The listing builds one solid part. Answer for the finished solid, in the listing's coordinates (mm). Face numbers are marked on the shaded views. A direction names the side the tool comes from. Round coordinates to 2 decimals unless told otherwise and drop trailing zeros. Loops run counter-clockwise (first coordinate to the right, second up) from the corner with the lowest first, then second, coordinate; pieces in that order, holes last. Notation, with made-up numbers: (65, -37) -> (105, -37) arc R6 cw to (105, -27) -> close; hole circle Ø5 at (59.25, 89.5). An arc over 180 degrees is marked (long way). Write each question's results on one line, items separated by ' | '. Start each with the question number.
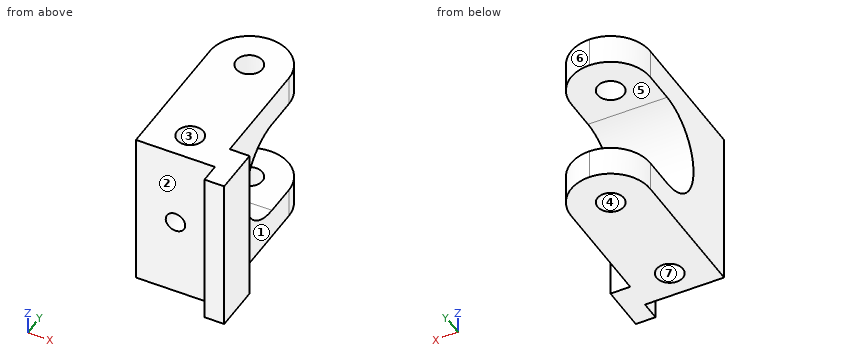
Autodesk Inventor part; units mm, degrees
ref_plane "YZ Plane" through (0, 0, 0) normal (1, 0, 0) x (0, 1, 0)
ref_plane "XZ Plane" through (0, 0, 0) normal (0, 1, 0) x (-1, 0, 0)
ref_plane "XY Plane" through (0, 0, 0) normal (0, 0, 1) x (1, 0, 0)
sketch "草圖1" plane through (0, 0, 0) normal (1, 0, 0) x (0, 1, 0)
  arc A0 (0, 12.5) -> (0, -12.5) centre (0, 0) ccw
  line L0 (-27, 0) -> (-27, -20)
  line L1 (-27, -20) -> (18, -20)
  line L2 (18, 20) -> (-27, 20)
  line L3 (-27, 20) -> (-27, 0)
  line L4 (0, 12.5) -> (18, 12.5)
  line L5 (18, -12.5) -> (0, -12.5)
  line L6 (18, -12.5) -> (18, -20)
  line L7 (18, 12.5) -> (18, 20)
  dimension "d5" = 25
  dimension "d12" = 18
  dimension "d13" = 45
  dimension "d15" = 40
  dimension "d16" = 45
  dimension "d17" = 7.5
  dimension "d18" = 7.5
  dimension "d19" = 18
extrude "擠出1" add sketch "草圖1" along normal mid plane 20
sketch "草圖2" plane through (-10, -27, 20) normal (0, 0, 1) x (1, 0, 0)
  line L0 (20, 0) -> (20, 45)
  line L1 (20, 0) -> (20, 7)
  line L2 (20, 7) -> (25, 7)
  line L3 (25, 7) -> (25, 0)
  line L4 (25, 0) -> (25, -5)
  line L5 (25, -5) -> (20, -5)
  line L6 (0, 0) -> (20, 0)
  line L7 (20, -5) -> (20, 0)
  point P0 (10, 27)
  dimension "d22" = 7
  dimension "d23" = 5
  dimension "d24" = 5
extrude "擠出2" add sketch "草圖2" against normal up to surface (40 mm away)
fillet "圓角1" radius 10 4 edges at (10, 18, 16.25) (-10, 18, 16.25) (10, 18, -16.25) (-10, 18, -16.25)
sketch "草圖3" plane through (10, -32, 20) normal (0, 0, 1) x (1, 0, 0)
  line L0 (-20, 5) -> (0, 5)
  point P0 (-10, 32)
  point P1 (-10, 40)
  dimension "d30" = 35
hole "孔1" at (0, 8, 20) direction (0, 0, -1) diameter 6.647 end through all
sketch "草圖4" plane through (10, -32, 20) normal (0, 0, 1) x (1, 0, 0)
  line L0 (-20, 5) -> (0, 5)
  point P0 (-10, 32)
  point P1 (-10, 12)
  dimension "d38" = 7
hole "孔2" at (0, -20, 20) direction (0, 0, -1) diameter 6.647 depth 12 tip angle 118
mirror "鏡射1" about plane through (0, 0, 0) normal (0, 0, 1) of "孔2"
sketch "草圖5" plane through (-10, -27, -20) normal (0, -1, 0) x (1, 0, 0)
  point P0 (10, 20)
  point P1 (10, 20)
hole "孔3" at (0, -27, 0) direction (0, 1, 0) diameter 4.917 depth 12 tip angle 118
properties part number "7. 砲座"
Item 1: The part is cut by section A-A, the plane y = -5.5. Give the vertices of the cut face in (x, z).
Item 2: For the marked faces 1, 2 and 3, determine the directions among +Z, -Z, +X, -X, +Y, -Y from which every point of the face is accessible in a straight line to the end or side of a thin tool.
Item 3: Determine the mould class of the marked faces 4, 5, 6 and 7 for opening direction X: +X half, -X half, draft (parallel to the pull), parting line (faces both ways), or undercut.
Item 4: The part is cut by section C-C, the plane x = -7.25. Give the vertices of the cut face in (y, z).
Item 5: Straight lines are drawn through the part: L1, parallel to Y at x = 0, z = -16; L2, parallel to X at y = 8, z = -16.75; L3, parallel to Y at x = -1, z = 16. For each, find the intervals that lie inside material, in ascending order. Write a range as [from, to].
Item 6: The part is cut by section B-B, the plane z = 15.5. Give the number of separate pieces and of enclosed holes in the cut face, plus the area to 3 significant figures.
Item 7: Each of these flat-tipped pins is pushed along its axis until it touches: pin 1 Ø3 at (x, z) = (12.5, 11) entering from +Y; pin 2 Ø5 at (y, z) = (-11, -10) entering from +X; pin 3 Ø6 at (x, y) = (0, -20) entering from -Z. Where does it stop, or does it pass through?
Item 8: The part is cut by section D-D, the plane z = 7. Give the vertices of the cut face in (x, y), plus the area to 3 significant figures.
Report:
1) outline: (-10, -20) -> (10, -20) -> (10, -11.22) -> (-10, -11.22) -> close; (-10, 11.22) -> (10, 11.22) -> (10, 20) -> (-10, 20) -> close
2) face 1: +Z, -Z, +X, +Y | face 2: +Z, -Z, -X, -Y | face 3: +Z
3) face 4: undercut | face 5: draft | face 6: +X half | face 7: undercut
4) outline: (-27, -20) -> (14.89, -20) -> (14.89, -12.5) -> (0, -12.5) arc R12.5 cw to (0, 12.5) -> (14.89, 12.5) -> (14.89, 20) -> (-27, 20) -> close
5) L1: y = [-27, -23.32], [-16.68, 4.68], [11.32, 18] | L2: x = [-10, -3.32], [3.32, 10] | L3: y = [-27, -23.17], [-16.83, 4.83], [11.17, 17.95]
6) separate pieces: 1 | enclosed holes: 2 | area: 848 mm2
7) pin 1: stops at y = -20 | pin 2: stops at x = 10 | pin 3: stops at z = -7.81
8) outline: (-10, -27) -> (10, -27) -> (10, -32) -> (15, -32) -> (15, -20) -> (10, -20) -> (10, -10.36) -> (-10, -10.36) -> close; hole circle Ø3.32 at (0, -20) | area: 384 mm2
